from build123d import *

# Parameters (mm, degrees)
F3_DEPTH = 4
F4_SIZE  = 1
F5_SIZE  = 1


with BuildPart() as f1:
    # F0 (on Front) → F1 (revolve)
    with BuildSketch(Plane.XZ):
        Polygon((0, 14.656888), (0, 0), (35, 0), (35, 5), (10, 5), align=None)
    revolve(axis=Axis((41.428571, 0, 0), (1, 0, 0)))

    # F2 (on face) → F3 (cut)
    with BuildSketch(Plane(origin=(0, 0, 0), x_dir=(0, -1, 0), z_dir=(-1, 0, 0))):
        Polygon((-3.464102, -6), (3.464102, -6), (6.928203, 0), (3.464102, 6), (-3.464102, 6), (-6.928203, 0), align=None)
    extrude(amount=-F3_DEPTH, mode=Mode.SUBTRACT)

    # F4
    f4_edges = [f1.edges().sort_by_distance(p)[0] for p in [
        (35, 0, -5),
    ]]
    chamfer(f4_edges, length=F4_SIZE)

    # F5
    f5_edges = [f1.edges().sort_by_distance(p)[0] for p in [
        (0, 0, -14.656888),
    ]]
    chamfer(f5_edges, length=F5_SIZE)


solid = f1.part
Can you work these out from the model? Positions are in its coordinate system, mm. A direction names the side the tool comes from. Give positions to 0.01 mm unless a question says otherwise; leave off trailing zeros. Loops run counter-clockwise (first coordinate to the right, second up) from the corner with the lowest first, then second, coordinate; pieces in that order, holes last. Notation, with made-up numbers: (65, 83.25) -> (71, 83.25) arc R24 cw to (71, 108.25) -> close; hole circle Ø9 at (50, 33.5). An arc over 180 degrees is marked (long way). Return JSON: item names as keys, results as strings.
Q1. We'd pull the mould along Z, two halves only. Please class faces 4 (the face through (9.419, 5.428, -1.205)), 5 (the face through (0, -0.2, -6.3)), 6 (the face through (2, 0, 6)), 7 (the face through (1.97, 5.22, -2.96)): released by +Z, released by -Z, zero draft, split by the parting line, or undercut.
Checks:
{"face 4": "split by the parting line", "face 5": "zero draft", "face 6": "undercut", "face 7": "undercut"}
Q2. I want a section at A-A, the plane y = 0. List the corners of the cut face in (x, z) for me, then the cut area to 3 significant figures.
Checks:
{"outline": "(0, -13.66) -> (0.72, -13.96) -> (10, -5) -> (34, -5) -> (35, -4) -> (35, 4) -> (34, 5) -> (10, 5) -> (0.72, 13.96) -> (0, 13.66) -> (0, 6) -> (4, 6) -> (4, -6) -> (0, -6) -> close", "area": "397 mm2"}
Q3. I want a section at C-C, the plane x = 13. List the corners of the cut face in (y, z) for me, then the cut area to 3 significant figures.
Checks:
{"outline": "circle Ø10 at (0, 0)", "area": "78.5 mm2"}
Q4. I want a section at B-B, the plane x = 3. List the corners of the cut face in (y, z) for me, then the cut area to 3 significant figures.
Checks:
{"outline": "circle Ø23.52 at (0, 0); hole (-6.93, 0) -> (-3.46, -6) -> (3.46, -6) -> (6.93, 0) -> (3.46, 6) -> (-3.46, 6) -> close", "area": "310 mm2"}
Q5. I need wall thicknesses on probe 1 along X at (y, z) = (7, 3.75); probe 2 along X at (y, z) = (-1, 5.5); probe 3 along Y at (x, z) = (31, 4). Which ranges of each line are inside material? Lowest first, please.
Checks:
{"probe 1": "x = 0 to 6.95", "probe 2": "x = 4 to 9.39", "probe 3": "y = -3 to 3"}
Q6. For pin 1 Ø10 at (x, z) = (10, 9) entering from -Y; pin 2 Ø8 at (x, z) = (19.5, -11) entering from -Y; pin 3 Ø1.2 at (x, y) = (1.5, -1.5) entering from +Z; pin 4 Ø1.5 at (x, y) = (23.5, -3) entering from -Z, each with a flat end and sliding along its axis, tell me the tip position at first contact or that it passes through.
Checks:
{"pin 1": "stops at y = -6.53", "pin 2": "passes through", "pin 3": "stops at z = 13.71", "pin 4": "stops at z = -4.47"}
Q7. On a 3-axis mill with a long thin cutter (end or side, diameter ignored), from which of +Z, -Z, +X, -X, +Y, -Y can I reach the whole of each face in a straight line? I mean faces 1 (the face through (35, 0, 0)), 2 (the face through (21.83, 4.88, -1.08)), 3 (the face through (1.972, -5.172, -3.042)). Say none if no direction works.
Checks:
{"face 1": "+Z, -Z, +X, +Y, -Y", "face 2": "+X", "face 3": "-X"}
